Autodesk Inventor part; units mm, degrees
ref_plane "YZ Plane" through (0, 0, 0) normal (1, 0, 0) x (0, 1, 0)
ref_plane "XZ Plane" through (0, 0, 0) normal (0, 1, 0) x (-1, 0, 0)
ref_plane "XY Plane" through (0, 0, 0) normal (0, 0, 1) x (1, 0, 0)
sketch "Sketch1" plane through (0, 0, 0) normal (0, 0, 1) x (1, 0, 0)
  line L0 (7.62, 12.7) -> (-7.62, 12.7)
  line L1 (-7.62, 12.7) -> (-7.62, -12.7)
  line L2 (-7.62, -12.7) -> (7.62, -12.7)
  line L3 (7.62, -12.7) -> (7.62, 12.7)
  line L4 (7.62, 12.7) -> (-7.62, -12.7) construction
  line L5 (-7.62, 12.7) -> (7.62, -12.7) construction
  circle A0 centre (0, 0) radius 6.096
  circle A1 centre (0, -8.89) radius 1.524
  line L6 (7.62, 7.62) -> (-7.62, 7.62)
  point P0 (0, 7.62)
  dimension "d0" = 12.192
  dimension "d1" = 15.24
  dimension "d2" = 25.4
  dimension "d7" = 3.048
  dimension "d8" = 8.89
  dimension "d10" = 7.62
extrude "Extrusion1" add sketch "Sketch1" along normal blind 3.175 contours L3 L2 L1 L6 | A0
extrude "Extrusion2" add sketch "Sketch1" along normal blind 26.67 from surface at 3.175 contours A0
properties part number "FRONT_AXEL"
Source: CAD feature listing. Evaluate the final solid. Frame: model axes, mm. A direction names the side the tool comes from. Coordinates: 2 decimals unless noted, no trailing zeros. Write each loop counter-clockwise with the first axis right and the second up, starting at its lowest first coordinate (ties: lowest second). Pieces come first, ordered by that corner, then holes. Notation, with made-up numbers: (43.5, 12.5) -> (100.5, 12.5) arc R24 cw to (100.5, 41.5) -> close; hole circle Ø9 at (69, 56). An arc over 180 degrees is marked (long way). Return JSON: item names as keys, results as strings. Group by question number.
1) Ray query, line 1 along Y through (x, z) = (0, 1.55); line 2 along Z through (x, y) = (7.25, -5.75) (3 decimals); line 3 along X through (y, z) = (-0.25, 8.75). Return the intervals inside material, ascending.
2) Section query D-D, the plane y = 0. Return loops of the section in (x, z) (3 decimals).
3) Section query A-A, the plane y = -8.89. Return loops of the section in (x, z) (3 decimals), plus the area to 3 significant figures.
4) Section query C-C, the plane z = 11.5. Return loops of the section in (x, y), plus the area to 3 significant figures.
5) Mould query, pull axis Y, two halves, no side actions, for faces 3 (the face through (0, -7, 3.175)), 4 (the face through (0, 7.62, 2)), 5 (the face through (-0.33, -7.402, 1.565)), 6 (the face through (0, -12.7, 2)). Classes: +Y half, -Y half, draft (parallel to the pull), parting line (faces both ways), or undercut.
6) Set-up query: faces 1 (the face through (-0.794, -6.044, 16.323)), 2 (the face through (0, -2, 0)). Return all of +Z, -Z, +X, -X, +Y, -Y with unobstructed straight access to the full face (end or side cutting, diameter ignored); none if empty.
7) Contact query for flat-ended pins moving along their axis: P1, Ø1.5, axis at x = 1.5, z = 24, coming from the -Y side; P2, Ø2, axis at x = 0.5, z = 12.5, coming from the -Y side; P3, Ø10, axis at y = 3, z = 10, coming from the +X side. Output: stop coordinate, or through.
8) Section query B-B, the plane x = 0. Return loops of the section in (y, z) (3 decimals), plus the area to 3 significant figures.
From the geometry:
{
 "1": {"line 1": "-12.7 to -10.41, -7.37 to 7.62", "line 2": "0 to 3.175", "line 3": "-6.09 to 6.09"},
 "2": {"outline": "(-7.62, 0) -> (7.62, 0) -> (7.62, 3.175) -> (6.096, 3.175) -> (6.096, 29.845) -> (-6.096, 29.845) -> (-6.096, 3.175) -> (-7.62, 3.175) -> close"},
 "3": {"outline": "(-7.62, 0) -> (-1.524, 0) -> (-1.524, 3.175) -> (-7.62, 3.175) -> close; (1.524, 0) -> (7.62, 0) -> (7.62, 3.175) -> (1.524, 3.175) -> close", "area": "38.7 mm²"},
 "4": {"outline": "circle Ø12.19 at (0, 0)", "area": "117 mm²"},
 "5": {"face 3": "draft", "face 4": "+Y half", "face 5": "undercut", "face 6": "-Y half"},
 "6": {"face 1": "+Z", "face 2": "-Z, +X, -X, +Y, -Y"},
 "7": {"P1": "y = -6.05", "P2": "y = -6.1", "P3": "x = 6.1"},
 "8": {"outline": "(-12.7, 0) -> (-10.414, 0) -> (-10.414, 3.175) -> (-12.7, 3.175) -> close; (-7.366, 0) -> (7.62, 0) -> (7.62, 3.175) -> (6.096, 3.175) -> (6.096, 29.845) -> (-6.096, 29.845) -> (-6.096, 3.175) -> (-7.366, 3.175) -> close", "area": "380 mm²"}
}
